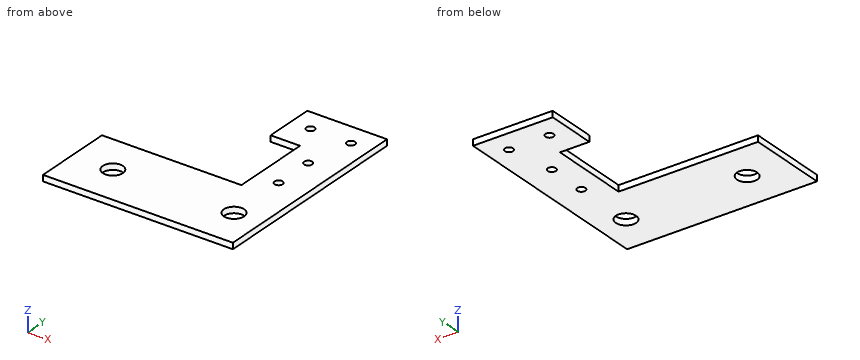
from build123d import *

# Parameters (mm, degrees)
SKETCH1_R           = 2.5
SKETCH1_R_2         = 1
BOSS_EXTRUDE1_DEPTH = 1.5


with BuildPart() as part:
    # Sketch1 → Boss-Extrude1 (new body)
    with BuildSketch(Plane.XY):
        Polygon((-19.743694785, 19.646203879), (-12.475339463, 19.646203879), (-12.475339463, -0.233517887), (-47.013694785, -0.233517887), (-47.013694785, -20.233517887), (0, -20.233517887), (0, 0), (0, 32.06155097), (-19.743694785, 32.06155097), align=None)
        with Locations((-37.013694785, -10.233517887)):
            Circle(SKETCH1_R, mode=Mode.SUBTRACT)
        with BuildLine():
            ThreePointArc((-4.513694785, -10.233517887), (-7.013694785, -12.733517887), (-9.513694785, -10.233517887))
            ThreePointArc((-9.513694785, -10.233517887), (-7.013694785, -7.733517887), (-4.513694785, -10.233517887))
        make_face(mode=Mode.SUBTRACT)
        with Locations((-7.013694785, 4.91155097)):
            Circle(SKETCH1_R_2, mode=Mode.SUBTRACT)
        with Locations((-7.013694785, 14.91155097)):
            Circle(SKETCH1_R_2, mode=Mode.SUBTRACT)
        with Locations((-14.873694785, 26.50155097)):
            Circle(SKETCH1_R_2, mode=Mode.SUBTRACT)
        with Locations((-4.873694785, 26.50155097)):
            Circle(SKETCH1_R_2, mode=Mode.SUBTRACT)
    extrude(amount=BOSS_EXTRUDE1_DEPTH)


solid = part.part
Check sheet for the modelled part. Datum: model origin and axes. Units: mm. Round coordinates to 2 decimals unless told otherwise and drop trailing zeros. Write each loop counter-clockwise with the first axis right and the second up, starting at its lowest first coordinate (ties: lowest second). Pieces come first, ordered by that corner, then holes. Notation, with made-up numbers: (-3.75, 75) - (47.25, 75) arc R25 cw to (47.25, 99) - close; hole circle Ø3 at (20, 27). An arc over 180 degrees is marked (long way). Return JSON: item names as keys, results as strings.
Q1. Cross-section at C-C (z = 0.55). Record the boundary of the cut face in (x, y), then the cut area to 3 significant figures.
Returned:
{"outline": "(-47.01, -20.23) - (0, -20.23) - (0, 32.06) - (-19.74, 32.06) - (-19.74, 19.65) - (-12.48, 19.65) - (-12.48, -0.23) - (-47.01, -0.23) - close; hole circle Ø5 at (-37.01, -10.23); hole circle Ø2 at (-14.87, 26.5); hole circle Ø5 at (-7.01, -10.23); hole circle Ø2 at (-7.01, 4.91); hole circle Ø2 at (-7.01, 14.91); hole circle Ø2 at (-4.87, 26.5)", "area": "1,380 mm²"}
Q2. Scan lines: L1, parallel to Y at x = -7, z = 0.35; L2, parallel to X at y = -11.5, z = 1.1; L3, parallel to X at y = -9.5, z = 0.9. Record each from-to range of solid material in increasing order. Write a range as from..to.
Returned:
{"L1": "y = -20.23..-12.73, -7.73..3.91, 5.91..13.91, 15.91..32.06", "L2": "x = -47.01..-39.17, -34.86..-9.17, -4.86..0", "L3": "x = -47.01..-39.4, -34.62..-9.4, -4.62..0"}
Q3. Cross-section at A-A (x = -37). Record the boundary of the cut face in (y, z).
Returned:
{"outline": "(-20.23, 0) - (-12.73, 0) - (-12.73, 1.5) - (-20.23, 1.5) - close; (-7.73, 0) - (-0.23, 0) - (-0.23, 1.5) - (-7.73, 1.5) - close"}
Q4. Cross-section at D-D (y = 23.5). Record the boundary of the cut face in (x, z), then the cut area to 3 significant figures.
Returned:
{"outline": "(-19.74, 0) - (0, 0) - (0, 1.5) - (-19.74, 1.5) - close", "area": "29.6 mm²"}
Q5. Depth check by flat-ended pin: P1, Ø12, axis at x = -32, y = 11, coming from the -Z side; P2, Ø0.8, axis at y = 28.5, z = 1, coming from the -X side. Enter the tip coordinate at first touch or a pass-through.
Returned:
{"P1": "passes through", "P2": "stops at x = -19.74"}
Q6. Cross-section at B-B (y = -8.5). Record the boundary of the cut face in (x, z).
Returned:
{"outline": "(-47.01, 0) - (-38.82, 0) - (-38.82, 1.5) - (-47.01, 1.5) - close; (-35.21, 0) - (-8.82, 0) - (-8.82, 1.5) - (-35.21, 1.5) - close; (-5.21, 0) - (0, 0) - (0, 1.5) - (-5.21, 1.5) - close"}
